The model under review builds one solid part; all positions refer to its coordinate system, in mm. Give positions to 0.01 mm unless a question says otherwise; leave off trailing zeros. Write each loop counter-clockwise with the first axis right and the second up, starting at its lowest first coordinate (ties: lowest second). Pieces come first, ordered by that corner, then holes.
from build123d import *

# Parameters (mm, degrees)
SKETCH_W                     = 15.24
SKETCH_H                     = 15.24
PAD_DEPTH                    = 1.6
SKETCH001_R                  = 0.51
POCKET_DEPTH                 = 44.824845
SKETCH001_LINEARPATTERN_2_R  = 0.51
POCKET_LINEARPATTERN_2_DEPTH = 44.824845
SKETCH001_LINEARPATTERN_3_R  = 0.51
POCKET_LINEARPATTERN_3_DEPTH = 44.824845
SKETCH001_LINEARPATTERN_4_R  = 0.51
POCKET_LINEARPATTERN_4_DEPTH = 44.824845
SKETCH001_LINEARPATTERN_5_R  = 0.51
POCKET_LINEARPATTERN_5_DEPTH = 44.824845
SKETCH001_LINEARPATTERN_6_R  = 0.51
POCKET_LINEARPATTERN_6_DEPTH = 44.824845
SKETCH001_LINEARPATTERN_7_R  = 0.51
POCKET_LINEARPATTERN_7_DEPTH = 44.824845
LINEARPATTERN003_COUNT       = 7
LINEARPATTERN003_PITCH       = 2.54


with BuildPart() as part:
    # Sketch → Pad (new body)
    with BuildSketch(Plane.XY):
        Rectangle(SKETCH_W, SKETCH_H)
    extrude(amount=PAD_DEPTH)

    # Sketch001 → Pocket (cut, through all)
    with BuildSketch(Plane.XY.offset(1.6)):
        with Locations((-7.62, 7.62)):
            Circle(SKETCH001_R)
    pocket = extrude(amount=-POCKET_DEPTH, mode=Mode.SUBTRACT)

    # Sketch001 LinearPattern 2 → Pocket LinearPattern 2 (cut, through all)
    with BuildSketch(Plane(origin=(2.54, 0, 1.6), x_dir=(1, 0, 0), z_dir=(0, 0, 1))):
        with Locations((-7.62, 7.62)):
            Circle(SKETCH001_LINEARPATTERN_2_R)
    pocket_linearpattern_2 = extrude(amount=-POCKET_LINEARPATTERN_2_DEPTH, mode=Mode.SUBTRACT)

    # Sketch001 LinearPattern 3 → Pocket LinearPattern 3 (cut, through all)
    with BuildSketch(Plane(origin=(5.08, 0, 1.6), x_dir=(1, 0, 0), z_dir=(0, 0, 1))):
        with Locations((-7.62, 7.62)):
            Circle(SKETCH001_LINEARPATTERN_3_R)
    pocket_linearpattern_3 = extrude(amount=-POCKET_LINEARPATTERN_3_DEPTH, mode=Mode.SUBTRACT)

    # Sketch001 LinearPattern 4 → Pocket LinearPattern 4 (cut, through all)
    with BuildSketch(Plane(origin=(7.62, 0, 1.6), x_dir=(1, 0, 0), z_dir=(0, 0, 1))):
        with Locations((-7.62, 7.62)):
            Circle(SKETCH001_LINEARPATTERN_4_R)
    pocket_linearpattern_4 = extrude(amount=-POCKET_LINEARPATTERN_4_DEPTH, mode=Mode.SUBTRACT)

    # Sketch001 LinearPattern 5 → Pocket LinearPattern 5 (cut, through all)
    with BuildSketch(Plane(origin=(10.16, 0, 1.6), x_dir=(1, 0, 0), z_dir=(0, 0, 1))):
        with Locations((-7.62, 7.62)):
            Circle(SKETCH001_LINEARPATTERN_5_R)
    pocket_linearpattern_5 = extrude(amount=-POCKET_LINEARPATTERN_5_DEPTH, mode=Mode.SUBTRACT)

    # Sketch001 LinearPattern 6 → Pocket LinearPattern 6 (cut, through all)
    with BuildSketch(Plane(origin=(12.7, 0, 1.6), x_dir=(1, 0, 0), z_dir=(0, 0, 1))):
        with Locations((-7.62, 7.62)):
            Circle(SKETCH001_LINEARPATTERN_6_R)
    pocket_linearpattern_6 = extrude(amount=-POCKET_LINEARPATTERN_6_DEPTH, mode=Mode.SUBTRACT)

    # Sketch001 LinearPattern 7 → Pocket LinearPattern 7 (cut, through all)
    with BuildSketch(Plane(origin=(15.24, 0, 1.6), x_dir=(1, 0, 0), z_dir=(0, 0, 1))):
        with Locations((-7.62, 7.62)):
            Circle(SKETCH001_LINEARPATTERN_7_R)
    pocket_linearpattern_7 = extrude(amount=-POCKET_LINEARPATTERN_7_DEPTH, mode=Mode.SUBTRACT)

    # LinearPattern003: Pocket, Pocket LinearPattern 2, Pocket LinearPattern 3, Pocket LinearPattern 4, Pocket LinearPattern 5, Pocket LinearPattern 6, Pocket LinearPattern 7 ×7
    with Locations(*[(0, -i * LINEARPATTERN003_PITCH, 0) for i in range(1, LINEARPATTERN003_COUNT)]):
        add(pocket, mode=Mode.SUBTRACT)
        add(pocket_linearpattern_2, mode=Mode.SUBTRACT)
        add(pocket_linearpattern_3, mode=Mode.SUBTRACT)
        add(pocket_linearpattern_4, mode=Mode.SUBTRACT)
        add(pocket_linearpattern_5, mode=Mode.SUBTRACT)
        add(pocket_linearpattern_6, mode=Mode.SUBTRACT)
        add(pocket_linearpattern_7, mode=Mode.SUBTRACT)


solid = part.part
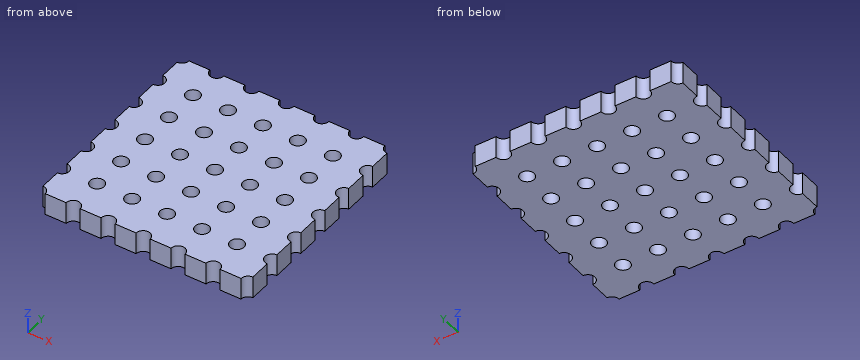
1) Consider section C-C, the plane z = 1.35. State how many separate pieces and enclosed holes the cut face has, then the cut area to 3 significant figures.
2) Insertion check: pin 1 (0.6 mm diameter, centred on x = -2.54, y = 0, fed in from -Z); pin 2 (1.3 mm diameter, centred on x = 5.08, y = 0, fed in from -Z). Each pin has a flat end and moves straight along its axis. Give the tip position at first contact, or say it passes through.
3) Consider section A-A, the plane y = 2.54. Give the boundary of the cut face in (x, z), then the cut area to 3 significant figures.
4) To check wall thickness, follow probe 1 along X at (y, z) = (2.5, 1.15); probe 2 along X at (y, z) = (-2.25, 0.7). State the ranges of each line that lie inside material, in increasing order.
Answer block:
1. separate pieces: 1
1. enclosed holes: 25
1. area: 203 mm2
2. pin 1: passes through
2. pin 2: stops at z = 0
3. outline: (-7.11, 0) - (-5.59, 0) - (-5.59, 1.6) - (-7.11, 1.6) - close; (-4.57, 0) - (-3.05, 0) - (-3.05, 1.6) - (-4.57, 1.6) - close; (-2.03, 0) - (-0.51, 0) - (-0.51, 1.6) - (-2.03, 1.6) - close; (0.51, 0) - (2.03, 0) - (2.03, 1.6) - (0.51, 1.6) - close; (3.05, 0) - (4.57, 0) - (4.57, 1.6) - (3.05, 1.6) - close; (5.59, 0) - (7.11, 0) - (7.11, 1.6) - (5.59, 1.6) - close
3. area: 14.6 mm2
4. probe 1: x = -7.11 to -5.59, -4.57 to -3.05, -2.03 to -0.51, 0.51 to 2.03, 3.05 to 4.57, 5.59 to 7.11
4. probe 2: x = -7.2 to -5.5, -4.66 to -2.96, -2.12 to -0.42, 0.42 to 2.12, 2.96 to 4.66, 5.5 to 7.2
